from build123d import *

# Parameters (mm, degrees)
F0_W     = 152.4
F0_H     = 114.3
F1_DEPTH = 12.7
F2_W     = 76.2
F2_H     = 114.3
F3_DEPTH = 79.248
F4_R     = 31.75
F5_DEPTH = 114.301


with BuildPart() as f1:
    # F0 (on Top) → F1 (new body)
    with BuildSketch(Plane.XY):
        with Locations((-30.01758, 19.292982)):
            Rectangle(F0_W, F0_H)
    extrude(amount=F1_DEPTH)

    # F2 (on face) → F3 (join)
    with BuildSketch(Plane.XY.offset(12.7)):
        with Locations((-30.01758, 19.292982)):
            Rectangle(F2_W, F2_H)
    extrude(amount=F3_DEPTH)

    # F4 (on face) → F5 (cut, through all)
    with BuildSketch(Plane.XZ.offset(37.857018)):
        with Locations((-30.01758, 91.948)):
            Circle(F4_R)
    extrude(amount=-F5_DEPTH, mode=Mode.SUBTRACT)


solid = f1.part
Geometry check sheet. Reference: the model listing, model coordinates, mm. A direction names the side the tool comes from. Round coordinates to 2 decimals unless told otherwise and drop trailing zeros. Order: outer loops, then holes, each group sorted by start corner. A loop starts at its lowest first (then second) coordinate and runs counter-clockwise, first axis right, second up. Notation, with made-up numbers: M 67.5,20 L 87.5,20 A16 ccw 87.5,35 Z; hole C 14,56 d2. An arc over 180 degrees is marked long. Answer in a Markdown table with one row per item. Add a question column.
Item 1: Set-up check for faces 1 (the face through (27, 20, 12.7)), 2 (the face through (-87, 20, 12.7)), 3 (the face through (-31, 76.443, 35)): record each of +Z, -Z, +X, -X, +Y, -Y from which the full face is reachable in a straight line by a thin tool's end or side.
Item 2: Sectioned sample at D-D, the plane z = 50.5. Enter the section's corners in (x, y), plus the area to 3 significant figures.
Item 3: Sectioned sample at C-C, the plane x = 11. Enter the section's corners in (y, z), plus the area to 3 significant figures.
Item 4: Material ranges on L1, parallel to Z at x = 18, y = -32; L2, parallel to X at y = 48, z = 44.5; L3, parallel to X at y = 70, z = 70.5, recorded low to high. Write a range as [from, to].
Item 5: Sectioned sample at A-A, the plane z = 76. Enter the section's corners in (x, y), plus the area to 3 significant figures.
Item 6: Depth check by flat-ended pin: pin 1 Ø11.5 at (x, y) = (33.5, 12) entering from +Z; pin 2 Ø1.5 at (y, z) = (22, 63) entering from +X; pin 3 Ø24 at (y, z) = (-4.5, 68) entering from -X. Enter the tip coordinate at first touch or a pass-through.
Item 7: Sectioned sample at B-B, the plane y = 52.5. Enter the section's corners in (x, z).
Filled in:
| question | item | result |
|---|---|---|
| 1 | face 1 | +Z, +X, +Y, -Y |
| 1 | face 2 | +Z, -X, +Y, -Y |
| 1 | face 3 | +Z, -Z, +X, -X, +Y |
| 2 | outline | M -68.12,-37.86 L 8.08,-37.86 L 8.08,76.44 L -68.12,76.44 Z |
| 2 | area | 8,710 mm² |
| 3 | outline | M -37.86,0 L 76.44,0 L 76.44,12.7 L -37.86,12.7 Z |
| 3 | area | 1,450 mm² |
| 4 | L1 | z = [0, 12.7] |
| 4 | L2 | x = [-68.12, 8.08] |
| 4 | L3 | x = [-68.12, -53.43], [-6.61, 8.08] |
| 5 | outline | M -68.12,-37.86 L -57.47,-37.86 L -57.47,76.44 L -68.12,76.44 Z; M -2.56,-37.86 L 8.08,-37.86 L 8.08,76.44 L -2.56,76.44 Z |
| 5 | area | 2,430 mm² |
| 6 | pin 1 | stops at z = 12.7 |
| 6 | pin 2 | stops at x = 8.08 |
| 6 | pin 3 | stops at x = -68.12 |
| 7 | outline | M -106.22,0 L 46.18,0 L 46.18,12.7 L 8.08,12.7 L 8.08,91.95 L 1.73,91.95 A31.75 cw -61.77,91.95 L -68.12,91.95 L -68.12,12.7 L -106.22,12.7 Z |
